The model under review builds one solid part; all positions refer to its coordinate system, in mm. A direction names the side the tool comes from. Coordinates: 2 decimals unless noted, no trailing zeros. Order: outer loops, then holes, each group sorted by start corner. A loop starts at its lowest first (then second) coordinate and runs counter-clockwise, first axis right, second up. Notation, with made-up numbers: M 40,-17.75 L 51,-17.75 A7 ccw 51,-4.75 Z; hole C -14.5,-36 d5. An arc over 180 degrees is marked long. Answer in a Markdown table with one row per item.
from build123d import *

# Parameters (mm, degrees)
BOSS_EXTRUDE1_DEPTH = 15
CUT_EXTRUDE5_REACH  = 43.908
SKETCH9_R           = 2
CUT_EXTRUDE6_REACH  = 43.908
SKETCH10_R          = 2
CUT_EXTRUDE7_REACH  = 40.079
FILLET1_R           = 0.5
CUT_EXTRUDE8_REACH  = 39.141
SKETCH11_R          = 3.5
CUT_EXTRUDE9_REACH  = 39.141
SKETCH12_R          = 3.5


with BuildPart() as part:
    # Sketch1 → Boss-Extrude1 (new body)
    with BuildSketch(Plane(origin=(0, 0, 0), x_dir=(1, 0, 0), z_dir=(0, 1, 0))):
        Polygon((-24.748737342, 0), (24.748737342, 0), (0, -24.748737342), align=None)
    extrude(amount=BOSS_EXTRUDE1_DEPTH)

    # Cut-Extrude5: up to this plane
    cut_extrude5_end = Plane(origin=(-24.748737342, 15, 0), z_dir=(0, 0, 1))
    # Sketch9 → Cut-Extrude5 (cut, up to the surface)
    with BuildSketch(Plane(origin=(12.374368671, 0, 12.374368671), x_dir=(0.7071067811865474, 0, -0.7071067811865477), z_dir=(0.7071067811865477, 0, 0.7071067811865474)), mode=Mode.PRIVATE) as cut_extrude5_sk1:
        with Locations((-6.75, 7.5)):
            Circle(SKETCH9_R)
    cut_extrude5_tool1 = split(extrude(cut_extrude5_sk1.sketch, amount=-CUT_EXTRUDE5_REACH, mode=Mode.PRIVATE), bisect_by=cut_extrude5_end, keep=Keep.BOTH, mode=Mode.PRIVATE)
    add(cut_extrude5_tool1.solids().sort_by_distance((7.601398, 7.5, 17.147339))[0], mode=Mode.SUBTRACT)
    # Sketch9 → Cut-Extrude5 (cut, up to the surface)
    with BuildSketch(Plane(origin=(12.374368671, 0, 12.374368671), x_dir=(0.7071067811865474, 0, -0.7071067811865477), z_dir=(0.7071067811865477, 0, 0.7071067811865474)), mode=Mode.PRIVATE) as cut_extrude5_sk2:
        with Locations((6.75, 7.5)):
            Circle(SKETCH9_R)
    cut_extrude5_tool2 = split(extrude(cut_extrude5_sk2.sketch, amount=-CUT_EXTRUDE5_REACH, mode=Mode.PRIVATE), bisect_by=cut_extrude5_end, keep=Keep.BOTH, mode=Mode.PRIVATE)
    add(cut_extrude5_tool2.solids().sort_by_distance((17.147339, 7.5, 7.601398))[0], mode=Mode.SUBTRACT)

    # Cut-Extrude6: up to this plane
    cut_extrude6_end = Plane(origin=(-24.748737342, 15, 0), z_dir=(0, 0, 1))
    # Sketch10 → Cut-Extrude6 (cut, up to the surface)
    with BuildSketch(Plane(origin=(-12.374368671, 0, 12.374368671), x_dir=(0.7071067811865472, 0, 0.7071067811865479), z_dir=(-0.7071067811865479, 0, 0.7071067811865472)), mode=Mode.PRIVATE) as cut_extrude6_sk1:
        with Locations((-6.75, 7.5)):
            Circle(SKETCH10_R)
    cut_extrude6_tool1 = split(extrude(cut_extrude6_sk1.sketch, amount=-CUT_EXTRUDE6_REACH, mode=Mode.PRIVATE), bisect_by=cut_extrude6_end, keep=Keep.BOTH, mode=Mode.PRIVATE)
    add(cut_extrude6_tool1.solids().sort_by_distance((-17.147339, 7.5, 7.601398))[0], mode=Mode.SUBTRACT)
    # Sketch10 → Cut-Extrude6 (cut, up to the surface)
    with BuildSketch(Plane(origin=(-12.374368671, 0, 12.374368671), x_dir=(0.7071067811865472, 0, 0.7071067811865479), z_dir=(-0.7071067811865479, 0, 0.7071067811865472)), mode=Mode.PRIVATE) as cut_extrude6_sk2:
        with Locations(Location((6.75, 7.5, 0), (0, 0, 90))):
            Circle(SKETCH10_R)
    cut_extrude6_tool2 = split(extrude(cut_extrude6_sk2.sketch, amount=-CUT_EXTRUDE6_REACH, mode=Mode.PRIVATE), bisect_by=cut_extrude6_end, keep=Keep.BOTH, mode=Mode.PRIVATE)
    add(cut_extrude6_tool2.solids().sort_by_distance((-7.601398, 7.5, 17.147339))[0], mode=Mode.SUBTRACT)

    # Sketch3 → Cut-Extrude7 (cut, up to next)
    with BuildSketch(Plane.XZ, mode=Mode.PRIVATE) as cut_extrude7_sk1:
        Polygon((-2.5, 22.248737342), (0, 24.748737342), (2.5, 22.248737342), align=None)
    cut_extrude7_tool1 = extrude(cut_extrude7_sk1.sketch, amount=-CUT_EXTRUDE7_REACH, mode=Mode.PRIVATE) & part.part
    # Sketch3 → Cut-Extrude7 (cut, up to next)
    with BuildSketch(Plane.XZ, mode=Mode.PRIVATE) as cut_extrude7_sk2:
        Polygon((-24.748737342, 0), (-22.980970389, 1.767766953), (-21.213203436, 0), align=None)
    cut_extrude7_tool2 = extrude(cut_extrude7_sk2.sketch, amount=-CUT_EXTRUDE7_REACH, mode=Mode.PRIVATE) & part.part
    # Sketch3 → Cut-Extrude7 (cut, up to next)
    with BuildSketch(Plane.XZ, mode=Mode.PRIVATE) as cut_extrude7_sk3:
        Polygon((24.748737342, 0), (21.213203436, 0), (22.980970389, 1.767766953), align=None)
    cut_extrude7_tool3 = extrude(cut_extrude7_sk3.sketch, amount=-CUT_EXTRUDE7_REACH, mode=Mode.PRIVATE) & part.part
    add(cut_extrude7_tool1.solids().sort_by_distance((0, 0, 23.082071))[0], mode=Mode.SUBTRACT)
    add(cut_extrude7_tool2.solids().sort_by_distance((-22.98097, 0, 0.589256))[0], mode=Mode.SUBTRACT)
    add(cut_extrude7_tool3.solids().sort_by_distance((22.98097, 0, 0.589256))[0], mode=Mode.SUBTRACT)

    # Fillet1
    fillet1_edges = [part.edges().sort_by_distance(p)[0] for p in [
        (-12.740485194, 0, 12.008252147),
        (12.740485194, 0, 12.008252147),
        (-12.740485194, 15, 12.008252147),
        (12.740485194, 15, 12.008252147),
        (22.980970389, 7.5, 1.767766953),
        (22.097086912, 15, 0.883883476),
        (22.097086912, 0, 0.883883476),
        (-22.097086912, 15, 0.883883476),
        (-22.980970389, 7.5, 1.767766953),
        (-22.097086912, 0, 0.883883476),
    ]]
    fillet(fillet1_edges, radius=FILLET1_R)

    # Cut-Extrude8: up to this plane
    cut_extrude8_end = Plane(origin=(-24.748737342, 15, 0), z_dir=(0, 0, 1))
    # Sketch11 → Cut-Extrude8 (cut, up to the surface)
    with BuildSketch(Plane(origin=(-8.131727984, 0, 8.131727984), x_dir=(0.7071067811865475, 0, 0.7071067811865477), z_dir=(-0.7071067811865477, 0, 0.7071067811865475)), mode=Mode.PRIVATE) as cut_extrude8_sk1:
        with Locations((-6.75, 7.5)):
            Circle(SKETCH11_R)
    cut_extrude8_tool1 = split(extrude(cut_extrude8_sk1.sketch, amount=-CUT_EXTRUDE8_REACH, mode=Mode.PRIVATE), bisect_by=cut_extrude8_end, keep=Keep.BOTH, mode=Mode.PRIVATE)
    add(cut_extrude8_tool1.solids().sort_by_distance((-12.904699, 7.5, 3.358757))[0], mode=Mode.SUBTRACT)
    # Sketch11 → Cut-Extrude8 (cut, up to the surface)
    with BuildSketch(Plane(origin=(-8.131727984, 0, 8.131727984), x_dir=(0.7071067811865475, 0, 0.7071067811865477), z_dir=(-0.7071067811865477, 0, 0.7071067811865475)), mode=Mode.PRIVATE) as cut_extrude8_sk2:
        with Locations((6.75, 7.5)):
            Circle(SKETCH11_R)
    cut_extrude8_tool2 = split(extrude(cut_extrude8_sk2.sketch, amount=-CUT_EXTRUDE8_REACH, mode=Mode.PRIVATE), bisect_by=cut_extrude8_end, keep=Keep.BOTH, mode=Mode.PRIVATE)
    add(cut_extrude8_tool2.solids().sort_by_distance((-3.358757, 7.5, 12.904699))[0], mode=Mode.SUBTRACT)

    # Cut-Extrude9: up to this plane
    cut_extrude9_end = Plane(origin=(-24.748737342, 15, 0), z_dir=(0, 0, 1))
    # Sketch12 → Cut-Extrude9 (cut, up to the surface)
    with BuildSketch(Plane(origin=(8.131727984, 0, 8.131727984), x_dir=(0.7071067811865474, 0, -0.7071067811865477), z_dir=(0.7071067811865477, 0, 0.7071067811865474)), mode=Mode.PRIVATE) as cut_extrude9_sk1:
        with Locations((6.75, 7.5)):
            Circle(SKETCH12_R)
    cut_extrude9_tool1 = split(extrude(cut_extrude9_sk1.sketch, amount=-CUT_EXTRUDE9_REACH, mode=Mode.PRIVATE), bisect_by=cut_extrude9_end, keep=Keep.BOTH, mode=Mode.PRIVATE)
    add(cut_extrude9_tool1.solids().sort_by_distance((12.904699, 7.5, 3.358757))[0], mode=Mode.SUBTRACT)
    # Sketch12 → Cut-Extrude9 (cut, up to the surface)
    with BuildSketch(Plane(origin=(8.131727984, 0, 8.131727984), x_dir=(0.7071067811865474, 0, -0.7071067811865477), z_dir=(0.7071067811865477, 0, 0.7071067811865474)), mode=Mode.PRIVATE) as cut_extrude9_sk2:
        with Locations(Location((-6.75, 7.5, 0), (0, 0, 90))):
            Circle(SKETCH12_R)
    cut_extrude9_tool2 = split(extrude(cut_extrude9_sk2.sketch, amount=-CUT_EXTRUDE9_REACH, mode=Mode.PRIVATE), bisect_by=cut_extrude9_end, keep=Keep.BOTH, mode=Mode.PRIVATE)
    add(cut_extrude9_tool2.solids().sort_by_distance((3.358757, 7.5, 12.904699))[0], mode=Mode.SUBTRACT)


solid = part.part
(1) To check wall thickness, follow line 1 (X direction, y = 9.5, z = 2); line 2 (Z direction, x = 5, y = 8.25); line 3 (X direction, y = 4.5, z = 8). State the ranges of each line that lie inside material, in increasing order. Write a range as [from, to].
Report:
| item | result |
|---|---|
| line 1 | [-22.72, -14.26], [-3.48, 3.48], [14.26, 22.72] |
| line 2 | [9.38, 9.71], [11.26, 11.92], [17.17, 19.75] |
| line 3 | [-16.75, -4.1], [4.1, 16.75] |
(2) The part is to be moulded in two halves that separate along Y. For faces 3 (the cylindrical face through (12.137, 0.143, 12.399)), 4 (the flat face through (-12.42, 7.4, 12.33)), 5 (the cylindrical face through (-15.24, 9.483, 5.326)), 6 (the cylindrical face through (-5.57, 5.5, 14.99)), say which applies: +Y half, -Y half, draft (parallel to the pull), parting line (faces both ways), or undercut.
Report:
| item | result |
|---|---|
| face 3 | -Y half |
| face 4 | draft |
| face 5 | undercut |
| face 6 | undercut |
(3) Machinability: for faces 1 (the flat face through (0, 15, 8)), 2 (the flat face through (-1.743, 7.549, 14.52)), which of the approach directions +Z, -Z, +X, -X, +Y, -Y give a long, thin tool a straight path to every point of the face, cutting with its end or side? Answer none if there is none.
Report:
| item | result |
|---|---|
| face 1 | +Z, -Z, +X, -X, +Y |
| face 2 | none |
(4) Take a section at C-C (y = 8.75). State how many separate pieces and enclosed holes the cut face has, then the cut area to 3 significant figures.
Report:
| item | result |
|---|---|
| separate pieces | 6 |
| enclosed holes | 0 |
| area | 310 mm^2 |
(5) Take a section at B-B (y = 1.5). Write out the cut boundary in (x, z), then the cut area to 3 significant figures.
Report:
| item | result |
|---|---|
| outline | M -22.63,1.41 L -21.21,0 L 21.21,0 L 22.63,1.41 A0.5 ccw 22.63,2.12 L 2.5,22.25 L -2.5,22.25 L -22.63,2.12 A0.5 ccw Z |
| area | 600 mm^2 |
(6) Insertion check: P1, Ø2, axis at x = -15.5, y = 4.5, coming from the +Z side; P2, Ø1.5, axis at y = 8.5, z = 9.5, coming from the +X side; P3, Ø3, axis at x = 14.5, y = 5, coming from the +Z side. Each pin has a flat end and moves straight along its axis. Give the tip position at first contact, or say it passes through.
Report:
| item | result |
|---|---|
| P1 | z = 10.25 |
| P2 | x = 15.99 |
| P3 | z = 11.75 |
(7) Take a section at A-A (y = 5). Write out the cut boundary in (x, z), then the cut area to 3 significant figures.
Report:
| item | result |
|---|---|
| outline | M -22.63,1.41 L -21.21,0 L -13.01,0 L -14.64,1.63 L -11.17,5.09 L -9.55,3.46 L -3.46,9.55 L -5.09,11.17 L -1.63,14.64 L 0,13.01 L 1.63,14.64 L 5.09,11.17 L 3.46,9.55 L 9.55,3.46 L 11.17,5.09 L 14.64,1.63 L 13.01,0 L 21.21,0 L 22.63,1.41 A0.5 ccw 22.63,2.12 L 2.5,22.25 L -2.5,22.25 L -22.63,2.12 A0.5 ccw Z; M -6.08,0 L 6.08,0 L 0,6.08 Z |
| area | 423 mm^2 |
